Can you work these out from the model? Positions are in its coordinate system, mm. A direction names the side the tool comes from. Round coordinates to 2 decimals unless told otherwise and drop trailing zeros. Loops run counter-clockwise (first coordinate to the right, second up) from the corner with the lowest first, then second, coordinate; pieces in that order, holes last. Notation, with made-up numbers: (45, 33) -> (70, 33) arc R30 cw to (70, 68) -> close; hole circle Ø9 at (-30.75, -22). An arc over 180 degrees is marked (long way). Write item = value, one per line.
from build123d import *

# Parameters (mm, degrees)
SKETCH1_R           = 2.5
BOSS_EXTRUDE1_DEPTH = 3


with BuildPart() as part:
    # Sketch1 → Boss-Extrude1 (new body)
    with BuildSketch(Plane.XY):
        with BuildLine():
            Line((34.37, 75.95596391), (-15.63, 75.95596391))
            Line((-15.63, 75.95596391), (-15.63, 78.95596391))
            Line((-15.63, 78.95596391), (-41.63, 78.95596391))
            Line((-41.63, 78.95596391), (-41.63, 75.95596391))
            Line((-41.63, 75.95596391), (-46.697493122, 67.335029306))
            Line((-46.697493122, 67.335029306), (-49.283773504, 68.855277242))
            Line((-49.283773504, 68.855277242), (-56.885013187, 55.923875336))
            Line((-56.885013187, 55.923875336), (-54.298732806, 54.403627399))
            Line((-54.298732806, 54.403627399), (-60.44, 43.95596391))
            Line((-60.44, 43.95596391), (-63.44, 43.95596391))
            Line((-63.44, 43.95596391), (-63.44, 3.95596391))
            Line((-63.44, 3.95596391), (-60.44, 3.95596391))
            Line((-60.44, 3.95596391), (-60.44, -36.04403609))
            Line((-60.44, -36.04403609), (-63.44, -36.04403609))
            Line((-63.44, -36.04403609), (-63.44, -76.04403609))
            Line((-63.44, -76.04403609), (-60.44, -76.04403609))
            Line((-60.44, -76.04403609), (-15.324347337, -76.04403609))
            Line((-15.324347337, -76.04403609), (-15.324347337, -36.04403609))
            ThreePointArc((-15.324347337, -36.04403609), (0.56, -20.159688753), (16.444347337, -36.04403609))
            Line((16.444347337, -36.04403609), (16.444347337, -76.04403609))
            Line((16.444347337, -76.04403609), (60.37, -76.04403609))
            Line((60.37, -76.04403609), (60.37, 75.95596391))
            Line((60.37, 75.95596391), (60.37, 78.95596391))
            Line((60.37, 78.95596391), (34.37, 78.95596391))
            Line((34.37, 78.95596391), (34.37, 75.95596391))
        make_face()
        with Locations((-40.44, -66.04403609)):
            Circle(SKETCH1_R, mode=Mode.SUBTRACT)
        with Locations((40.37, -66.04403609)):
            Circle(SKETCH1_R, mode=Mode.SUBTRACT)
    extrude(amount=BOSS_EXTRUDE1_DEPTH)


solid = part.part
1. Suppose I cut it at A-A, the plane x = 40.37. List the corners of the cut face in (y, z) for me.
Entries:
outline = (-76.04, 0) -> (-68.54, 0) -> (-68.54, 3) -> (-76.04, 3) -> close; (-63.54, 0) -> (78.96, 0) -> (78.96, 3) -> (-63.54, 3) -> close
2. We'd pull the mould along Y, two halves only. Please class faces 1 (the flat face through (34.37, 77, 1)), 2 (the cylindrical face through (-40.982, -68.485, 1.479)), 3 (the flat face through (-57.3, 49.3, 1.5)), 4 (the flat face through (38, -76.044, 1)): released by +Y, released by -Y, zero draft, split by the parting line, or undercut.
Entries:
face_1 = zero draft
face_2 = undercut
face_3 = undercut
face_4 = released by -Y
3. Suppose I cut it at D-D, the plane x = 0.56. List the corners of the cut face in (y, z) for me, and give its area (3 significant figures).
Entries:
outline = (-20.16, 0) -> (75.96, 0) -> (75.96, 3) -> (-20.16, 3) -> close
area = 288 mm²
4. Suppose I cut it at B-B, the plane y = -34. List the corners of the cut face in (x, z) for me.
Entries:
outline = (-60.44, 0) -> (-15.19, 0) -> (-15.19, 3) -> (-60.44, 3) -> close; (16.31, 0) -> (60.37, 0) -> (60.37, 3) -> (16.31, 3) -> close
5. I need wall thicknesses on line 1 (X direction, y = -48, z = 2.1); line 2 (Y direction, x = 40.37, z = 1.65); line 3 (X direction, y = -23.5, z = 0.9). Which ranges of each line are inside material? Lowest first, please. Write a range as [from, to].
Entries:
line_1 = [-63.44, -15.32], [16.44, 60.37]
line_2 = [-76.04, -68.54], [-63.54, 78.96]
line_3 = [-60.44, -9.18], [10.3, 60.37]
6. For faces 5 (the flat face through (-53.03, 62.48, 1.48)), 6 (the flat face through (-15.63, 77, 1)), 7 (the flat face through (-62, 3.956, 1)), 8 (the flat face through (-63.44, -56, 1)), 9 (the flat face through (16.444, -56, 1)), which set-ups out of +Z, -Z, +X, -X, +Y, -Y let a thin tool reach every point of the face, with its end or its side?
Entries:
face_5 = +Z, -Z, -X, +Y
face_6 = +Z, -Z, +Y
face_7 = +Z, -Z, -X
face_8 = +Z, -Z, -X, +Y, -Y
face_9 = +Z, -Z, -Y
7. Suppose I cut it at C-C, the plane z = 1. List the corners of the cut face in (x, y) for me.
Entries:
outline = (-63.44, -76.04) -> (-15.32, -76.04) -> (-15.32, -36.04) arc R15.88 cw to (16.44, -36.04) -> (16.44, -76.04) -> (60.37, -76.04) -> (60.37, 78.96) -> (34.37, 78.96) -> (34.37, 75.96) -> (-15.63, 75.96) -> (-15.63, 78.96) -> (-41.63, 78.96) -> (-41.63, 75.96) -> (-46.7, 67.34) -> (-49.28, 68.86) -> (-56.89, 55.92) -> (-54.3, 54.4) -> (-60.44, 43.96) -> (-63.44, 43.96) -> (-63.44, 3.96) -> (-60.44, 3.96) -> (-60.44, -36.04) -> (-63.44, -36.04) -> close; hole circle Ø5 at (-40.44, -66.04); hole circle Ø5 at (40.37, -66.04)
8. I'm going to push flat-ended pins straight in: pin 1 (0.9 mm diameter, centred on x = -61.5, z = 1, fed in from +Y); pin 2 (4.5 mm diameter, centred on x = 40.37, y = -66.04, fed in from +Z); pin 3 (1.5 mm diameter, centred on y = 77, z = 2, fed in from -X); pin 4 (0.9 mm diameter, centred on x = 2.5, z = 1.5, fed in from +Y). Where does each tip first touch, or does it pass through?
Entries:
pin_1 = 43.96
pin_2 = through
pin_3 = -41.63
pin_4 = 75.96
